Can you work these out from the model? Positions are in its coordinate system, mm. A direction names the side the tool comes from. Give positions to 0.01 mm unless a question says otherwise; leave off trailing zeros. Return JSON: item names as keys, results as strings. Group by question number.
Q1. Thinking about a two-plate mould opening in X: for faces 1 (the flat face through (-0.14, -4.056, 8.864)), 2 (the flat face through (-10, 0, 5)), 3 (the cylindrical face through (-0.81, -5.7, -5.87)), 4 (the conical face through (0.2, 12.3, 5.5)), which applies, pulls with the +X half, pulls with the -X half, needs draft (parallel to the pull), parting line crosses it, or undercut?
Q2. Which directions (+Z, -Z, +X, -X, +Y, -Y) give clear straight access to the entire face, cutting with the end or side of a thin tool? Please do faces 5 (the flat face through (10.2, -3.4, 0)), 6 (the flat face through (2, 4.4, -20)), 7 (the flat face through (10, 0, 5)), 8 (the flat face through (-11, 0, 3)).
Q3. I need wall thicknesses on line 1 along X through (y, z) = (-5.25, -11); line 2 along Y through (x, z) = (1, -7.25); line 3 along Y through (x, z) = (5.5, -18). Which ranges of each line are inside material? Lowest first, please. Write a range as [from, to].
Q4. Will these pins go through, and if not, where does the flat tip stop? pin 1 (5 mm diameter, centred on x = 5, z = -15, fed in from +Y); pin 2 (4 mm diameter, centred on x = -2.5, y = -2, fed in from +Z); pin 3 (8 mm diameter, centred on y = -3.5, z = -12.5, fed in from +X) (3 decimals).
```python
from build123d import *

# Parameters (mm, degrees)
F0_R           = 10.525
F1_DEPTH       = 20
F3_R           = 12.5
F4_DEPTH       = 10
F5_SIZE2       = 5
F5_SIZE        = 2
F8_SIZE        = 1
F9_R           = 0.5
F12_R          = 6.25
F13_DEPTH      = 29.8925289631
F13_DEPTH_BACK = 3.9949082022
F14_W          = 35.6293991208
F14_H          = 33.7468273938
F15_DEPTH      = 3.9949082022
F16_R          = 0.5
F18_W          = 42.0981385947
F18_H          = 52.5076624169
F18_W_2        = 21.5321744272
F18_H_2        = 55.8203060705
F19_DEPTH      = 6.9380379737
F20_R          = 1


with BuildPart() as f1:
    # F0 (on Top) → F1 (new body)
    with BuildSketch(Plane.XY):
        Circle(F0_R)
    extrude(amount=-F1_DEPTH)

    # F3 (on face) → F4 (join)
    with BuildSketch(Plane.XY):
        Circle(F3_R)
    extrude(amount=F4_DEPTH)

    # F5
    f5_edges = [f1.edges().sort_by_distance(p)[0] for p in [
        (-12.5, 0, 10),
    ]]
    f5_side = f1.faces().sort_by_distance((0, 0, 10))[0]
    chamfer(f5_edges, length=F5_SIZE, length2=F5_SIZE2, reference=f5_side)

    # F8
    f8_edges = [f1.edges().sort_by_distance(p)[0] for p in [
        (-12.5, 0, 0),
    ]]
    chamfer(f8_edges, length=F8_SIZE)

    # F9
    f9_edges = [f1.edges().sort_by_distance(p)[0] for p in [
        (-12.5, 0, 5),
    ]]
    fillet(f9_edges, radius=F9_R)

    # F12 (on face) → F13 (cut, two sides)
    with BuildSketch(Plane(origin=(0, 1.3934869758, 7.9028573515), x_dir=(1, 0, 0), z_dir=(0, -0.1736481777, -0.984807753))) as f13_sk:
        with Locations((0, -1.60399963)):
            Circle(F12_R)
    extrude(amount=F13_DEPTH, mode=Mode.SUBTRACT)
    extrude(f13_sk.sketch, amount=-F13_DEPTH_BACK, mode=Mode.SUBTRACT)

    # F14 (on face) → F15 (cut, through all)
    with BuildSketch(Plane(origin=(0, 1.3934869758, 7.9028573515), x_dir=(1, 0, 0), z_dir=(0, -0.1736481777, -0.984807753))):
        with Locations((0.3942959011, 1.4900509268)):
            Rectangle(F14_W, F14_H)
    extrude(amount=-F15_DEPTH, mode=Mode.SUBTRACT)

    # F16
    f16_edges = [f1.edges().sort_by_distance(p)[0] for p in [
        (7.715975, -7.436279, 9.459783),
        (-7.715975, 9.029819, 6.556366),
    ]]
    fillet(f16_edges, radius=F16_R)

    # F18 (on offset) → F19 (cut, through all)
    with BuildSketch(Plane(origin=(0, 0, 3), x_dir=(1, 0, 0), z_dir=(0, 0, -1))):
        with Locations((31.0490692973, 0)):
            Rectangle(F18_W, F18_H)
        with Locations((-20.7660872136, 0)):
            Rectangle(F18_W_2, F18_H_2)
    extrude(amount=-F19_DEPTH, mode=Mode.SUBTRACT)

    # F20
    f20_edges = [f1.edges().sort_by_distance(p)[0] for p in [
        (-10.525, 0, -20),
    ]]
    fillet(f20_edges, radius=F20_R)


solid = f1.part
```
Ans:
{
 "1": {"face 1": "needs draft", "face 2": "pulls with the -X half", "face 3": "undercut", "face 4": "parting line crosses it"},
 "2": {"face 5": "-Z", "face 6": "-Z, +X, -X, +Y, -Y", "face 7": "+Z, +X, +Y, -Y", "face 8": "+Z, -X, +Y, -Y"},
 "3": {"line 1": "x = [-9.12, -3.92], [3.92, 9.12]", "line 2": "y = [-10.48, -5.91], [6.62, 10.48]", "line 3": "y = [-8.97, -4.56], [1.47, 8.97]"},
 "4": {"pin 1": "stops at y = 10.22", "pin 2": "stops at z = 8.85", "pin 3": "stops at x = 10.525"}
}
